Geometry check sheet. Reference: the model listing, model coordinates, mm. A direction names the side the tool comes from. Give positions to 0.01 mm unless a question says otherwise; leave off trailing zeros. Order: outer loops, then holes, each group sorted by start corner. A loop starts at its lowest first (then second) coordinate and runs counter-clockwise, first axis right, second up. Notation, with made-up numbers: M 29.25,31 L 64.25,31 A20 cw 64.25,70 Z; hole C -6,-36 d10. An arc over 180 degrees is marked long. Answer as a JSON object with one key per item and string values. Group by question number.
from build123d import *

# Parameters (mm, degrees)
SLOPED_COVER_BLANK_DEPTH                        = 95
SLOPED_COVER_BLANK_DEPTH_BACK                   = 95
OPEN_BOTTOM_AND_FRONT_COVER_CAVITY_DEPTH        = 80
OPEN_BOTTOM_AND_FRONT_COVER_CAVITY_DEPTH_BACK   = 80
F_12_MM_FULL_LENGTH_SHAPE_DEFINING_ROOF_CH_SIZE = 12


with BuildPart() as part:
    # Sloped Cover Outer Side Profile → Sloped Cover Blank (new, two sides: drawn at the far end of the back side and taken through both)
    with BuildSketch(Plane(origin=(0, 0, 0), x_dir=(0, 0, -1), z_dir=(1, 0, 0)).offset(-SLOPED_COVER_BLANK_DEPTH_BACK)):
        Polygon((-22, 25), (-22, 200), (-60, 200), (-108, 60), (-108, 35), align=None)
    extrude(amount=SLOPED_COVER_BLANK_DEPTH + SLOPED_COVER_BLANK_DEPTH_BACK)

    # Open Bottom Cover Cavity Profile → Open Bottom and Front Cover Cavity (cut, two sides: drawn at the far end of the back side and taken through both)
    with BuildSketch(Plane(origin=(0, 0, 0), x_dir=(0, 0, -1), z_dir=(1, 0, 0)).offset(-OPEN_BOTTOM_AND_FRONT_COVER_CAVITY_DEPTH_BACK)):
        Polygon((-18, 23), (-18, 193), (-48, 193), (-96, 60), (-96, 33.604651163), align=None)
    extrude(amount=OPEN_BOTTOM_AND_FRONT_COVER_CAVITY_DEPTH + OPEN_BOTTOM_AND_FRONT_COVER_CAVITY_DEPTH_BACK, mode=Mode.SUBTRACT)

    # 12 mm Full-Length Shape-Defining Roof Chamfers
    f_12_mm_full_length_shape_defining_roof_ch_edges = [part.edges().sort_by_distance(p)[0] for p in [
        (95, 130, 84),
        (95, 47.5, 108),
        (-95, 130, 84),
        (-95, 47.5, 108),
    ]]
    chamfer(f_12_mm_full_length_shape_defining_roof_ch_edges, length=F_12_MM_FULL_LENGTH_SHAPE_DEFINING_ROOF_CH_SIZE)


solid = part.part
1. Cross-section at A-A (y = 54.5). Record the cut outline in (x, z).
2. Cross-section at D-D (z = 100). Record the cut outline in (x, y).
3. Cross-section at C-C (x = -11.5). Record the cut outline in (y, z).
4. Access from +Z, -Z, +X, -X, +Y, -Y to the whole of each face (thin tool, end or side, straight path). Record for faces 1 (the flat face through (-7.48, 33.727, 97.053)), 2 (the flat face through (80, 92, 51)).
5. Release check for a two-part mould opening along X. For faces 3 (the flat face through (-1, 48, 108)), 4 (the flat face through (-95, 94, 51)), 5 (the flat face through (-1, 47, 96)) record: released by +X, released by -X, zero draft, split by the parting line, or undercut.
6. Depth check by flat-ended pin: pin 1 (1.5 mm diameter, centred on x = 47, y = 101, fed in from +Z); pin 2 (1.5 mm diameter, centred on x = 73, z = 35, fed in from -Y); pin 3 (10 mm diameter, centred on x = -3.5, y = 169.5, fed in from -Z). Enter the tip coordinate at first touch or a pass-through.
7. Cross-section at B-B (z = 78). Record the cut outline in (x, y) (3 decimals).
8. Thickness scan on line 1 along X through (y, z) = (64, 69.5); line 2 along Y through (x, z) = (45.5, 45); line 3 along Z through (x, y) = (-62, 40). Record the ranges inside material, lowest first. Write a range as [from, to].
Report:
{
 "1": {"outline": "M -95,22 L -80,22 L -80,96 L 80,96 L 80,22 L 95,22 L 95,96 L 83,108 L -83,108 L -95,96 Z"},
 "2": {"outline": "M -91,34.07 L 91,34.07 L 91,58.67 L 83,83.33 L -83,83.33 L -91,58.67 Z"},
 "3": {"outline": "M 33.6,96 L 60,96 L 193,48 L 193,22 L 200,22 L 200,60 L 60,108 L 35,108 Z"},
 "4": {"face 1": "+Z, +X, -X, -Y", "face 2": "-Z, -Y"},
 "5": {"face 3": "zero draft", "face 4": "released by -X", "face 5": "undercut"},
 "6": {"pin 1": "stops at z = 94.2", "pin 2": "stops at y = 193", "pin 3": "stops at z = 54.68"},
 "7": {"outline": "M -95,31.512 L -80,31.512 L -80,109.875 L 80,109.875 L 80,31.512 L 95,31.512 L 95,110.5 L 83,147.5 L -83,147.5 L -95,110.5 Z"},
 "8": {"line 1": "x = [-95, -80], [80, 95]", "line 2": "y = [193, 200]", "line 3": "z = [96, 108]"}
}
